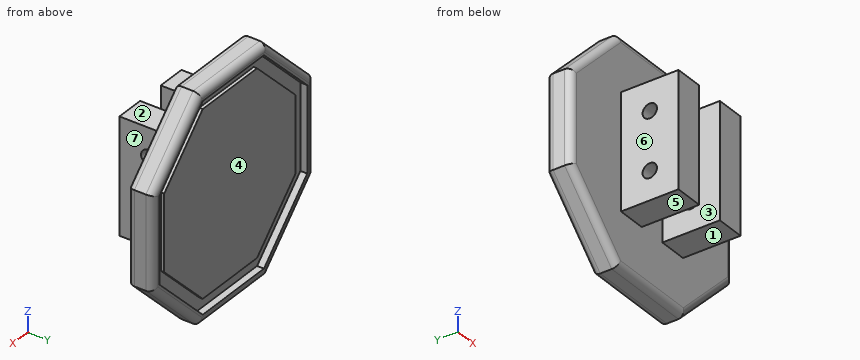
Autodesk Inventor part; units mm, degrees
ref_plane "YZ Plane" through (0, 0, 0) normal (1, 0, 0) x (0, 1, 0)
ref_plane "XZ Plane" through (0, 0, 0) normal (0, 1, 0) x (-1, 0, 0)
ref_plane "XY Plane" through (0, 0, 0) normal (0, 0, 1) x (1, 0, 0)
sketch "스케치3" plane through (0, 0, 0) normal (0, 1, 0) x (-1, 0, 0)
  line L0 (19.4959, -8.0755) -> (8.0755, -19.4959)
  line L1 (8.0755, -19.4959) -> (-8.0755, -19.4959)
  line L2 (-8.0755, -19.4959) -> (-19.4959, -8.0755)
  line L3 (-19.4959, -8.0755) -> (-19.4959, 8.0755)
  line L4 (-19.4959, 8.0755) -> (-8.0755, 19.4959)
  line L5 (-8.0755, 19.4959) -> (8.0755, 19.4959)
  line L6 (8.0755, 19.4959) -> (19.4959, 8.0755)
  line L7 (19.4959, 8.0755) -> (19.4959, -8.0755)
  line L8 (6.75, -16.2959) -> (-6.75, -16.2959)
  line L9 (-6.75, -16.2959) -> (-16.2959, -6.75)
  line L10 (-16.2959, -6.75) -> (-16.2959, 6.75)
  line L11 (-16.2959, 6.75) -> (-6.75, 16.2959)
  line L12 (-6.75, 16.2959) -> (6.75, 16.2959)
  line L13 (6.75, 16.2959) -> (16.2959, 6.75)
  line L14 (16.2959, 6.75) -> (16.2959, -6.75)
  line L15 (16.2959, -6.75) -> (6.75, -16.2959)
  point P0 (0, 0)
  point P1 (0, 0)
  point P2 (0, 0)
  point P3 (0, 0)
  dimension "d66" = 13.5
  dimension "d67" = 3.2
extrude "돌출2" add sketch "스케치3" along normal blind 4.4 contours L0 L1 L2 L3 L4 L5 L6 L7 | L8 L9 L10 L11 L12 L13 L14 L15
sketch "스케치9" plane through (0, 0, 0) normal (0, -1, 0) x (1, 0, 0)
  line L0 (7.5, 10) -> (2.5, 10)
  line L1 (2.5, 10) -> (2.5, -10)
  line L2 (2.5, -10) -> (7.5, -10)
  line L3 (7.5, -10) -> (7.5, 10)
  line L4 (7.5, 10) -> (2.5, -10) construction
  line L5 (2.5, 10) -> (7.5, -10) construction
  line L6 (-2.5, 10) -> (-7.5, 10)
  line L7 (-7.5, 10) -> (-7.5, -10)
  line L8 (-7.5, -10) -> (-2.5, -10)
  line L9 (-2.5, 10) -> (-7.5, -10) construction
  line L10 (-7.5, 10) -> (-2.5, -10) construction
  line L11 (-2.5, -10) -> (-2.5, 10)
  point P0 (0, 0)
  point P1 (5, 0)
  point P2 (-5, 0)
  dimension "d42" = 20
  dimension "d43" = 5
  dimension "d44" = 2.5
  dimension "d47" = 10
extrude "돌출8" add sketch "스케치9" along normal blind 10
sketch "스케치10" plane through (-7.5, 0, -10) normal (-1, 0, 0) x (0, 0, 1)
  circle A0 centre (15, -5) radius 1.25
  line L0 (19.9591, 0) -> (0.0886, 0)
  line L1 (18.0755, 0) -> (1.9245, 0)
  circle A1 centre (5, -5) radius 1.25
  line L2 (20, 0) -> (20, -10)
  point P0 (10, 0)
  dimension "d54" = 2.5
  dimension "d57" = 10
  dimension "d62" = 5
  dimension "d63" = 5
extrude "돌출9" cut sketch "스케치10" against normal blind 20
fillet "모깎기1" radius 1.2 16 edges at (-13.7857, 4.4, 13.7857) (0, 4.4, 19.4959) (13.7857, 4.4, 13.7857) (19.4959, 4.4, 0) (13.7857, 4.4, -13.7857) (0, 4.4, -19.4959) (-13.7857, 4.4, -13.7857) (-19.4959, 4.4, 0) (-13.7857, 0, 13.7857) (0, 0, 19.4959) (13.7857, 0, 13.7857) (19.4959, 0, 0) (13.7857, 0, -13.7857) (0, 0, -19.4959) (-13.7857, 0, -13.7857) (-19.4959, 0, 0)
sketch "스케치12" plane through (0, 4.4, 0) normal (0, 1, 0) x (1, 0, 0)
  line L0 (7.4127, -17.8959) -> (-7.4127, -17.8959)
  line L1 (-7.4127, -17.8959) -> (-17.8959, -7.4127)
  line L2 (-17.8959, -7.4127) -> (-17.8959, 7.4127)
  line L3 (-17.8959, 7.4127) -> (-7.4127, 17.8959)
  line L4 (-7.4127, 17.8959) -> (7.4127, 17.8959)
  line L5 (7.4127, 17.8959) -> (17.8959, 7.4127)
  line L6 (17.8959, 7.4127) -> (17.8959, -7.4127)
  line L7 (17.8959, -7.4127) -> (7.4127, -17.8959)
  line L8 (-6.5843, 15.8959) -> (6.5843, 15.8959)
  line L9 (6.5843, 15.8959) -> (15.8959, 6.5843)
  line L10 (15.8959, 6.5843) -> (15.8959, -6.5843)
  line L11 (15.8959, -6.5843) -> (6.5843, -15.8959)
  line L12 (6.5843, -15.8959) -> (-6.5843, -15.8959)
  line L13 (-6.5843, -15.8959) -> (-15.8959, -6.5843)
  line L14 (-15.8959, -6.5843) -> (-15.8959, 6.5843)
  line L15 (-15.8959, 6.5843) -> (-6.5843, 15.8959)
  line L16 (-18.2959, -7.5784) -> (-18.2959, 7.5784)
  line L17 (-19.4959, 8.0755) -> (-19.4959, -8.0755)
  point P0 (0, 0)
  point P1 (0, 0)
  point P2 (0, 0)
  point P3 (-17.8959, 0)
  point P4 (-19.4959, 0)
  point P5 (-15.8959, 0)
  dimension "d100" = 1.6
  dimension "d101" = 2
extrude "돌출11" cut sketch "스케치12" against normal blind 1.2
sketch "스케치13" plane through (0, 4.4, 0) normal (0, 1, 0) x (1, 0, 0)
  line L0 (15.8959, 6.5843) -> (6.5843, 15.8959)
  line L1 (6.5843, 15.8959) -> (-6.5843, 15.8959)
  line L2 (-6.5843, 15.8959) -> (-15.8959, 6.5843)
  line L3 (-15.8959, 6.5843) -> (-15.8959, -6.5843)
  line L4 (-15.8959, -6.5843) -> (-6.5843, -15.8959)
  line L5 (-6.5843, -15.8959) -> (6.5843, -15.8959)
  line L6 (6.5843, -15.8959) -> (15.8959, -6.5843)
  line L7 (15.8959, -6.5843) -> (15.8959, 6.5843)
  point P0 (0, 0)
extrude "돌출12" cut sketch "스케치13" against normal blind 0.6
properties part number "OV-PAM_bottom_2"
Source: CAD feature listing. Evaluate the final solid. Frame: model axes, mm. Face numbers are marked on the shaded views. A direction names the side the tool comes from. Coordinates: 2 decimals unless noted, no trailing zeros. Order: outer loops, then holes, each group sorted by start corner. A loop starts at its lowest first (then second) coordinate and runs counter-clockwise, first axis right, second up.
Item 1: Cut plane B-B (y = -3). Return loops of the section in (x, z).
Output values:
outline: (-7.5, -10) - (-2.5, -10) - (-2.5, 10) - (-7.5, 10) - close; (2.5, -10) - (7.5, -10) - (7.5, 10) - (2.5, 10) - close
Item 2: Cut plane C-C (y = -5.75). Return loops of the section in (x, z).
Output values:
outline: (-7.5, -10) - (-2.5, -10) - (-2.5, -6) - (-7.5, -6) - close; (-7.5, -4) - (-2.5, -4) - (-2.5, 4) - (-7.5, 4) - close; (-7.5, 6) - (-2.5, 6) - (-2.5, 10) - (-7.5, 10) - close; (2.5, -10) - (7.5, -10) - (7.5, -6) - (2.5, -6) - close; (2.5, -4) - (7.5, -4) - (7.5, 4) - (2.5, 4) - close; (2.5, 6) - (7.5, 6) - (7.5, 10) - (2.5, 10) - close
Item 3: Pull-direction query (X, two-part tool) for the marked faces 4, 5, 6 and 7; classes: pulls with the +X half, pulls with the -X half, needs draft (parallel to the pull), parting line crosses it, or undercut.
Output values:
face 4: undercut
face 5: needs draft
face 6: pulls with the -X half
face 7: pulls with the +X half
Item 4: First-contact query: P1, Ø3, axis at y = -5, z = 5, coming from the +X side; P2, Ø4, axis at x = -6, y = -3, coming from the -Z side; P3, Ø1, axis at x = -0.5, y = 4, coming from the +Z side. Flat tips, straight axial feed; report the tip coordinate or a pass-through.
Output values:
P1: stops at x = 7.5
P2: stops at z = -10
P3: stops at z = 19.46
Item 5: Material intervals for line 1 (Y direction, x = 5, z = -5); line 2 (X direction, y = -1.5, z = 2.5); line 3 (X direction, y = 3.5, z = 8), sorted ascending.
Output values:
line 1: y = -10 to -6.25, -3.75 to 3.8
line 2: x = -7.5 to -2.5, 2.5 to 7.5
line 3: x = -19.46 to -17.31, -14.48 to 14.48, 17.31 to 19.46
Item 6: Set-up query: the marked faces 1, 2 and 3. Return all of +Z, -Z, +X, -X, +Y, -Y with unobstructed straight access to the full face (end or side cutting, diameter ignored); none if empty.
Output values:
face 1: -Z, +X, -X, -Y
face 2: +Z, +X, -X, -Y
face 3: +Z, -Z, -Y
Item 7: Cut plane D-D (x = -3). Return loops of the section in (y, z), plus the area to 3 significant figures.
Output values:
outline: (-10, -10) - (0, -10) - (0, -18.3) arc R1.2 ccw to (1.2, -19.5) - (3.2, -19.5) arc R1.2 ccw to (4.4, -18.3) - (4.4, -17.9) - (3.2, -17.9) - (3.2, -15.9) - (3.8, -15.9) - (3.8, 15.9) - (3.2, 15.9) - (3.2, 17.9) - (4.4, 17.9) - (4.4, 18.3) arc R1.2 ccw to (3.2, 19.5) - (1.2, 19.5) arc R1.2 ccw to (0, 18.3) - (0, 10) - (-10, 10) - close; hole circle Ø2.5 at (-5, -5); hole circle Ø2.5 at (-5, 5)
area: 337 mm2
Item 8: Cut plane A-A (z = 5). Count the separate pieces of the cut face and the enclosed holes in it, plus the area to 3 significant figures.
Output values:
separate pieces: 3
enclosed holes: 0
area: 221 mm2
